```python
from build123d import *

# Parameters (mm, degrees)
PAD_DEPTH = 1


with BuildPart() as part:
    # Sketch → Pad (new body, symmetric)
    with BuildSketch(Plane.XZ):
        with BuildLine():
            Line((-15, -12), (4.5, -12))
            Line((4.5, -10.45), (4.5, -12))
            Line((6.2, -10.45), (4.5, -10.45))
            Line((6.2, -12), (6.2, -10.45))
            Line((6.2, -12), (9, -12))
            Line((9, -12), (9, 2))
            Line((-5.9714, 2), (9, 2))
            ThreePointArc((-5.9714, 4), (-9.70345, 3), (-5.9714, 2))
            Line((9, 4), (-5.9714, 4))
            Line((9, 12), (9, 4))
            Line((9, 12), (5.3, 12))
            Line((5.3, 7), (5.3, 12))
            Line((1.5, 7), (5.3, 7))
            Line((1.5, 12), (1.5, 7))
            Line((1.5, 12), (-15, 12))
            ThreePointArc((-15, 12), (-27, 0), (-15, -12))
        make_face()
    extrude(amount=PAD_DEPTH, both=True)


solid = part.part
```
Build history of the part. All positions in model axes, mm. A direction names the side the tool comes from. Give positions to 0.01 mm unless a question says otherwise; leave off trailing zeros. Loops run counter-clockwise (first coordinate to the right, second up) from the corner with the lowest first, then second, coordinate; pieces in that order, holes last.
Item 1: Slice it at B-B, the plane y = -0.1. List the corners of the cut face in (x, z), and give its area (3 significant figures).
Answers follow:
outline: (-15, -12) - (4.5, -12) - (4.5, -10.45) - (6.2, -10.45) - (6.2, -12) - (9, -12) - (9, 2) - (-5.97, 2) arc R2 cw (long way) to (-5.97, 4) - (9, 4) - (9, 12) - (5.3, 12) - (5.3, 7) - (1.5, 7) - (1.5, 12) - (-15, 12) arc R12 ccw to start
area: 738 mm2
Item 2: Which spindle directions (+Z, -Z, +X, -X, +Y, -Y) get a long thin tool onto all of the face, cutting with end or side? Do faces 4 (the face through (3, 0, 7)), 5 (the face through (2, 0, 4)), 6 (the face through (5, 0, -10.45)). Say none if no direction does.
Answers follow:
face 4: +Z, +Y, -Y
face 5: +X, +Y, -Y
face 6: -Z, +Y, -Y
Item 3: Flat gauge pins, fed straight in: pin 1 (0.8 mm diameter, centred on x = 5, y = 0.5, fed in from -Z); pin 2 (1 mm diameter, centred on y = 0.5, z = 10.5, fed in from -X); pin 3 (1.2 mm diameter, centred on y = 0.5, z = -11.5, fed in from -X); pin 4 (2.5 mm diameter, centred on x = -7.7, z = 3, fed in from +Y). Where does each tip first touch, or does it go through?
Answers follow:
pin 1: stops at z = -10.45
pin 2: stops at x = -21.63
pin 3: stops at x = -20.02
pin 4: passes through
Item 4: Slice it at C-C, the plane x = -19.5. List the corners of the cut face in (y, z).
Answers follow:
outline: (-1, -11.12) - (1, -11.12) - (1, 11.12) - (-1, 11.12) - close
Item 5: Slice it at A-A, the plane x = -5. List the corners of the cut face in (y, z).
Answers follow:
outline: (-1, -12) - (1, -12) - (1, 2) - (-1, 2) - close; (-1, 4) - (1, 4) - (1, 12) - (-1, 12) - close
Item 6: Pull direction X, two halves, no side cores. Call faces 1 (the face through (4.5, 0, -11)), 2 (the face through (8, 0, -12)), 3 (the face through (-27, 0, 0)): released by +X, released by -X, zero draft, split by the parting line, or undercut.
Answers follow:
face 1: undercut
face 2: zero draft
face 3: released by -X
Item 7: Slice it at D-D, the plane z = -4.25. List the corners of the cut face in (x, y), and give its area (3 significant figures).
Answers follow:
outline: (-26.22, -1) - (9, -1) - (9, 1) - (-26.22, 1) - close
area: 70.4 mm2
Item 8: Drill centre lines: line 1 (Z direction, x = -0.5, y = -0.1); line 2 (X direction, y = 0.5, z = 3); line 3 (Z direction, x = -17.5, y = -0.45). Where is each one in solid material? Low to high.
Answers follow:
line 1: z = -12 to 2, 4 to 12
line 2: x = -26.62 to -9.7
line 3: z = -11.74 to 11.74
